```python
from build123d import *

# Parameters (mm, degrees)
SKETCH1_W           = 13.9446
SKETCH1_H           = 13.8938
BOSS_EXTRUDE1_DEPTH = 1.27
SKETCH2_W           = 15.6464
SKETCH2_H           = 15.875
BOSS_EXTRUDE2_DEPTH = 1.016
SKETCH6_W           = 7.6454
SKETCH6_H           = 5.9944
BOSS_EXTRUDE4_DEPTH = 0.254
BOSS_EXTRUDE5_DEPTH = 3.556
SKETCH8_W           = 13.9446
SKETCH8_H           = 13.8938
BOSS_EXTRUDE6_DEPTH = 4.953
BOSS_EXTRUDE6_TAPER = 3


with BuildPart() as part:
    # Sketch1 → Boss-Extrude1 (new body)
    with BuildSketch(Plane(origin=(0, 0, 0), x_dir=(1, 0, 0), z_dir=(0, 1, 0))):
        Rectangle(SKETCH1_W, SKETCH1_H)
    extrude(amount=BOSS_EXTRUDE1_DEPTH)

    # Sketch2 → Boss-Extrude2 (add)
    with BuildSketch(Plane(origin=(0, 1.27, 0), x_dir=(1, 0, 0), z_dir=(0, 1, 0))):
        Rectangle(SKETCH2_W, SKETCH2_H)
    extrude(amount=BOSS_EXTRUDE2_DEPTH)

    # Sketch4 → Loft1 section 0
    with BuildSketch(Plane(origin=(0, 7.366, 0), x_dir=(1, 0, 0), z_dir=(0, 1, 0))):
        with BuildLine():
            Line((-5.0165, 5.5753), (5.0165, 5.5753))
            Line((5.0165, 5.5753), (5.0165, -3.8227))
            Line((5.0165, -3.8227), (-5.0165, -3.8227))
            Line((-5.0165, -3.8227), (-5.0165, 5.5753))
        make_face()
    # Sketch3 → Loft1 section 1
    with BuildSketch(Plane(origin=(0, 2.286, 0), x_dir=(1, 0, 0), z_dir=(0, 1, 0))):
        with BuildLine():
            Line((-7.2009, -7.3152), (7.2009, -7.3152))
            Line((7.2009, -7.3152), (7.2009, 7.3152))
            Line((7.2009, 7.3152), (-7.2009, 7.3152))
            Line((-7.2009, 7.3152), (-7.2009, -7.3152))
        make_face()
    loft()

    # Sketch6 → Boss-Extrude4 (add)
    with BuildSketch(Plane(origin=(0, 7.366, 0), x_dir=(1, 0, 0), z_dir=(0, 1, 0))):
        with Locations((0, 0.0889)):
            Rectangle(SKETCH6_W, SKETCH6_H)
    extrude(amount=BOSS_EXTRUDE4_DEPTH)

    # Sketch7 → Boss-Extrude5 (add)
    with BuildSketch(Plane(origin=(0, 7.62, 0), x_dir=(1, 0, 0), z_dir=(0, 1, 0))):
        Polygon((-0.5969, 0.5969), (-0.5969, 1.9685), (0.5969, 1.9685), (0.5969, 0.5969), (1.9685, 0.5969), (1.9685, -0.5969), (0.5969, -0.5969), (0.5969, -1.9685), (-0.5969, -1.9685), (-0.5969, -0.5969), (-1.9685, -0.5969), (-1.9685, 0.5969), align=None)
    extrude(amount=BOSS_EXTRUDE5_DEPTH)

    # Sketch8 → Boss-Extrude6 (add)
    with BuildSketch(Plane.XZ):
        Rectangle(SKETCH8_W, SKETCH8_H)
    extrude(amount=BOSS_EXTRUDE6_DEPTH, taper=BOSS_EXTRUDE6_TAPER)


solid = part.part
```
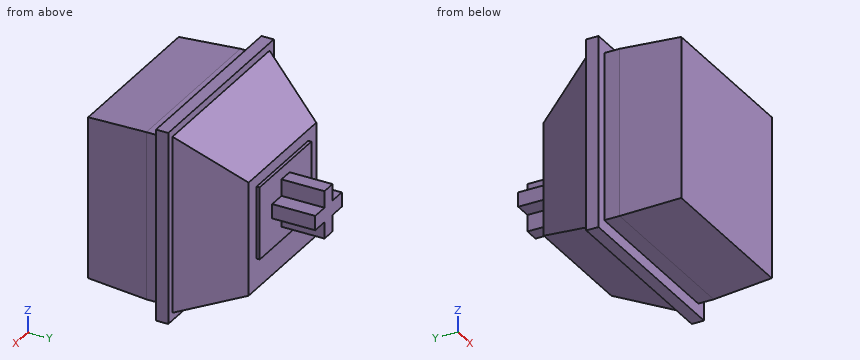
Model file for the job. Use its own axes, mm. Coordinates: 2 decimals unless noted, no trailing zeros. Loops run counter-clockwise (first coordinate to the right, second up) from the corner with the lowest first, then second, coordinate; pieces in that order, holes last. Notation, with made-up numbers: M 84,-16.5 L 123,-16.5 A11 cw 123,-12.5 Z; hole C 89.25,65.25 d5. An arc over 180 degrees is marked long. Use CSV: the item, a comma, the result in double quotes. Start each with the question number.
1. Band-saw the part on A-A, the plane y = 9.5. List the corners of the cut face in (x, z), then the cut area to 3 significant figures.
2. Flat gauge pins, fed straight in: pin 1 (1 mm diameter, centred on x = 3, y = 0.5, fed in from +Z); pin 2 (4 mm diameter, centred on x = 3, y = -1.5, fed in from -Z); pin 3 (8 mm diameter, centred on x = -5.5, z = -5.5, fed in from +Y). Where does each tip first touch, or does it go through?
3. Probe probe 1 along Y at (x, z) = (-1.75, 3.5); probe 2 along Z at (x, y) = (-0.25, 0.75); probe 3 along Y at (x, z) = (2.75, -1). List the from-to ranges inside material, lowest first. Write a range as [from, to].
Entries:
1,outline,"M -1.97,-0.6 L -0.6,-0.6 L -0.6,-1.97 L 0.6,-1.97 L 0.6,-0.6 L 1.97,-0.6 L 1.97,0.6 L 0.6,0.6 L 0.6,1.97 L -0.6,1.97 L -0.6,0.6 L -1.97,0.6 Z"
1,area,"7.97 mm2"
2,pin 1,"stops at z = 6.95"
2,pin 2,"stops at z = -6.95"
2,pin 3,"stops at y = 7.62"
3,probe 1,"y = [-4.95, 7.37]"
3,probe 2,"z = [-6.95, 6.95]"
3,probe 3,"y = [-4.95, 7.62]"
